Can you work these out from the drawing? Everything is in mm from the part's minimum corner. A direction names the side the tool comes from. Give positions to 0.01 mm unless a question says otherwise; leave off trailing zeros. Order: outer loops, then holes, each group sorted by start corner. A loop starts at its lowest first (then second) coordinate and runs counter-clockwise, first axis right, second up. Notation, with made-up numbers: (81.25, 77) - (117.25, 77) arc R12 ccw to (117.25, 90) - close; hole circle Ø5 at (-17.75, 86.5). An arc over 180 degrees is marked (long way). One line per question, with ' | ' between items.
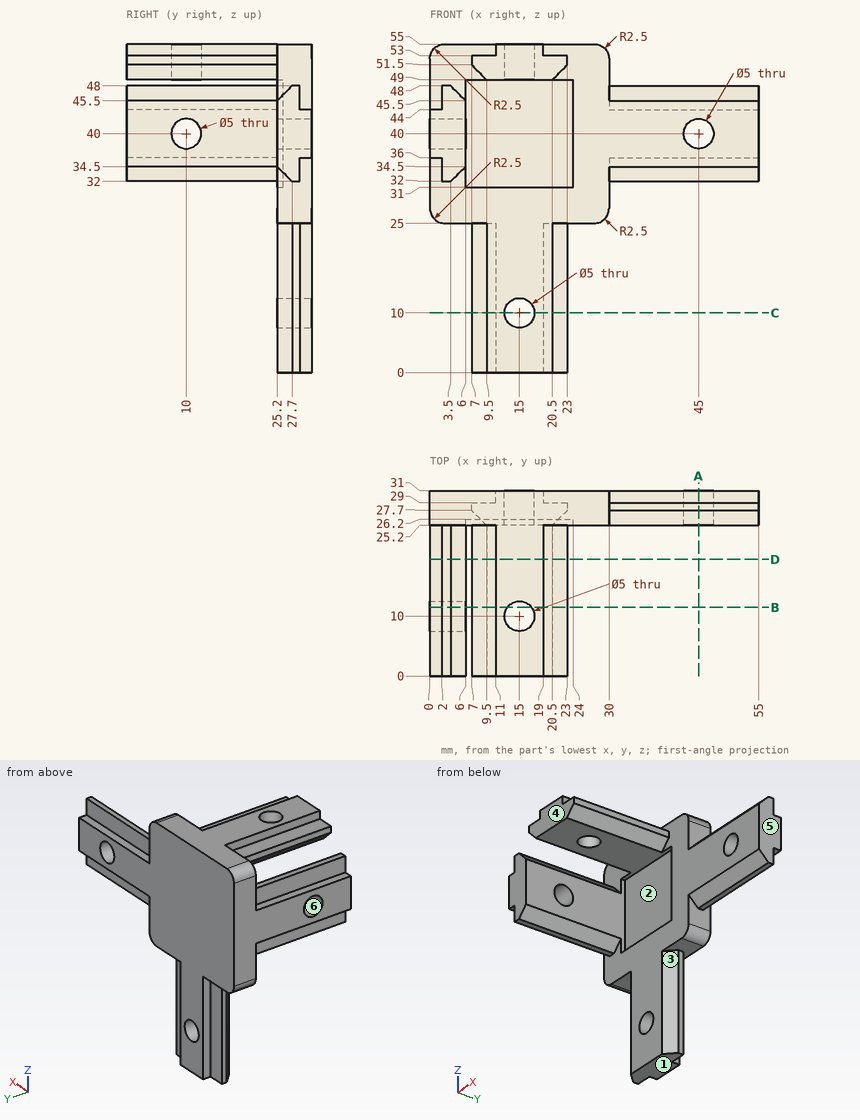
(1) Will these pins go through, and if not, where does the flat tip stop? pin 1 (1.2 mm diameter, centred on y = 18, z = 52.5, fed in from -X); pin 2 (0.6 mm diameter, centred on x = 42, y = 30, fed in from +Z); pin 3 (2 mm diameter, centred on x = 43.5, z = 45.5, fed in from +Y); pin 4 (3 mm diameter, centred on y = 10, z = 40, fed in from -X).
Answer below:
pin 1: x = 7 | pin 2: z = 44 | pin 3: y = 29 | pin 4: through
(2) If I drill on line 1 (Z direction, x = 15, y = 27.5); line 2 (X direction, y = 27.6, z = 40); line 3 (X direction, y = 28.45, z = 10), over which ranges is the centre line in solid material (lowest first)?
Answer below:
line 1: 0 to 7.5, 12.5 to 55 | line 2: 0 to 42.5, 47.5 to 55 | line 3: 7 to 12.5, 17.5 to 23
(3) Imagine slicing it at C-C (z = 10). List the corners of the cut face in (x, y) for me.
Answer below:
outline: (7, 27.7) - (9.5, 25.2) - (12.5, 25.2) - (12.5, 31) - (11, 31) - (11, 29) - (7, 29) - close; (17.5, 25.2) - (20.5, 25.2) - (23, 27.7) - (23, 29) - (19, 29) - (19, 31) - (17.5, 31) - close
(4) If we mould it in two halves opening along Y, with no side actions, what happens to the marked faces 4, 5 and 6? For each: released by +Y, released by -Y, zero draft, split by the parting line, or undercut.
Answer below:
face 4: released by -Y | face 5: zero draft | face 6: undercut
(5) Imagine slicing it at D-D (y = 19.5). List the corners of the cut face in (x, z) for me, and give its area (4 significant figures).
Answer below:
outline: (0, 36) - (2, 36) - (2, 32) - (3.5, 32) - (6, 34.5) - (6, 45.5) - (3.5, 48) - (2, 48) - (2, 44) - (0, 44) - close; (7, 51.5) - (9.5, 49) - (20.5, 49) - (23, 51.5) - (23, 53) - (19, 53) - (19, 55) - (11, 55) - (11, 53) - (7, 53) - close | area: 147.5 mm^2
(6) Imagine slicing it at A-A (x = 45). List the corners of the cut face in (y, z) for me, and give its area (4 significant figures).
Answer below:
outline: (25.2, 34.5) - (27.7, 32) - (29, 32) - (29, 36) - (31, 36) - (31, 37.5) - (25.2, 37.5) - close; (25.2, 42.5) - (31, 42.5) - (31, 44) - (29, 44) - (29, 48) - (27.7, 48) - (25.2, 45.5) - close | area: 41.55 mm^2
(7) On a 3-axis mill with a long thin cutter (end or side, diameter ignored), from which of +Z, -Z, +X, -X, +Y, -Y can I reach the whole of each face in a straight line? I mean the marked faces 1, 2 and 3. Say none if no direction works.
Answer below:
face 1: -Z, +X, -X, +Y, -Y | face 2: -Y | face 3: -Z, +X, -Y
(8) Imagine slicing it at B-B (y = 11.5). List the corners of the cut face in (x, z) for me.
Answer below:
outline: (0, 36) - (2, 36) - (2, 32) - (3.5, 32) - (6, 34.5) - (6, 38) - (0, 38) - close; (0, 42) - (6, 42) - (6, 45.5) - (3.5, 48) - (2, 48) - (2, 44) - (0, 44) - close; (7, 51.5) - (9.5, 49) - (13, 49) - (13, 55) - (11, 55) - (11, 53) - (7, 53) - close; (17, 49) - (20.5, 49) - (23, 51.5) - (23, 53) - (19, 53) - (19, 55) - (17, 55) - close
